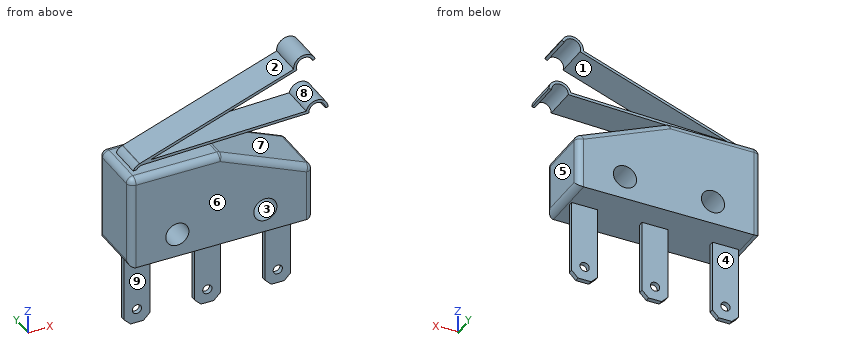
from build123d import *

# Parameters (mm, degrees)
F0_R     = 1.25
F1_DEPTH = 3.2
F2_R     = 0.7
F4_DEPTH = 1.8
F5_W     = 2.8
F5_H     = 9.0560415828
F5_R     = 0.5
F6_DEPTH = 0.25
F7_SIZE  = 0.7
F9_DEPTH = 3.6


with BuildPart() as f1:
    # F0 (on Front) → F1 (new body, symmetric)
    with BuildSketch(Plane.XZ):
        Polygon((-14.2658203304, 13.9623457611), (-24.1658203304, 13.9623457611), (-24.1658203304, 3.7623457611), (-4.3658203304, 3.7623457611), (-4.3658203304, 9.7123457611), align=None)
        with Locations((-19.0158203304, 6.2623457611)):
            Circle(F0_R, mode=Mode.SUBTRACT)
        with Locations((-9.5158203304, 6.2623457611)):
            Circle(F0_R, mode=Mode.SUBTRACT)
    extrude(amount=F1_DEPTH, both=True)

    # F2
    f2_edges = [f1.edges().sort_by_distance(p)[0] for p in [
        (-4.36582, 0, 9.712346),
        (-14.26582, 0, 13.962346),
        (-24.16582, 0, 13.962346),
        (-4.36582, 0, 3.762346),
        (-24.16582, 0, 3.762346),
        (-19.21582, -3.2, 13.962346),
        (-9.31582, -3.2, 11.837346),
        (-4.36582, -3.2, 6.737346),
        (-4.36582, 3.2, 6.737346),
        (-9.31582, 3.2, 11.837346),
        (-19.21582, 3.2, 13.962346),
        (-24.16582, -3.2, 8.862346),
        (-24.16582, 3.2, 8.862346),
    ]]
    fillet(f2_edges, radius=F2_R)

    # F3 (on Front) → F4 (join, symmetric)
    with BuildSketch(Plane.XZ):
        with BuildLine():
            Line((-4.3866957854, 15.2251207005), (-22.0158203304, 14.6623457611))
            ThreePointArc((-22.0158203304, 14.6623457611), (-23.165946247, 13.572328355), (-22.2182437598, 12.3023726214))
            Line((-22.2182437598, 12.3023726214), (-22.2182437598, 12.6108806694))
            ThreePointArc((-22.2182437598, 12.6108806694), (-22.8638430635, 13.5776541553), (-22.0062482997, 14.3624985062))
            Line((-22.0062482997, 14.3624985062), (-4.1153620949, 14.9336296691))
            ThreePointArc((-4.1153620949, 14.9336296691), (-3.2445364224, 15.8618875256), (-2.3162785659, 14.991061853))
            Line((-2.3162785659, 14.991061853), (-2.0164313111, 15.0006338837))
            ThreePointArc((-2.0164313111, 15.0006338837), (-3.1026751203, 16.1569997534), (-4.3866957854, 15.2251207005))
        make_face()
    extrude(amount=F4_DEPTH, both=True)

    # F5 (on Front) → F6 (join, symmetric)
    with BuildSketch(Plane.XZ):
        with Locations((-21.8658203304, -0.2096334475)):
            Rectangle(F5_W, F5_H)
        with Locations((-21.8658203304, -3.2376542389)):
            Circle(F5_R, mode=Mode.SUBTRACT)
        with Locations((-14.2658203304, -0.2096334475)):
            Rectangle(F5_W, F5_H)
        with Locations((-14.2658203304, -3.2376542389)):
            Circle(F5_R, mode=Mode.SUBTRACT)
        with Locations((-6.6658203304, -0.2096334475)):
            Rectangle(F5_W, F5_H)
        with Locations((-6.6658203304, -3.2376542389)):
            Circle(F5_R, mode=Mode.SUBTRACT)
    extrude(amount=F6_DEPTH, both=True)

    # F7
    f7_edges = [f1.edges().sort_by_distance(p)[0] for p in [
        (-12.86582, 0, -4.737654),
        (-15.66582, 0, -4.737654),
        (-20.46582, 0, -4.737654),
        (-23.26582, 0, -4.737654),
        (-5.26582, 0, -4.737654),
        (-8.06582, 0, -4.737654),
    ]]
    chamfer(f7_edges, length=F7_SIZE)

    # F8 (on face) → F9 (join, through all)
    with BuildSketch(Plane.XZ.offset(1.8)):
        with BuildLine():
            Line((-3.6950556462, 20.861555612), (-3.4121199517, 20.961292229))
            ThreePointArc((-3.4121199517, 20.961292229), (-4.7971701976, 21.7353058315), (-5.7393789628, 20.4587072715))
            Line((-5.7393789628, 20.4587072715), (-22.3494407238, 14.6035557305))
            Line((-22.3494407238, 14.6035557305), (-22.3988404472, 14.5861420164))
            ThreePointArc((-22.3988404472, 14.5861420164), (-23.1509491325, 13.2564048538), (-21.9777702725, 12.2778754681))
            Line((-21.9777702725, 12.2778754681), (-21.9777702725, 12.5778754681))
            ThreePointArc((-21.9777702725, 12.5778754681), (-22.8575253326, 13.319893669), (-22.2744995865, 14.3121844306))
            Line((-22.2744995865, 14.3121844306), (-5.3926698134, 20.2631359101))
            ThreePointArc((-5.3926698134, 20.2631359101), (-4.8430725807, 21.4111528446), (-3.6950556462, 20.861555612))
        make_face()
        with BuildLine():
            Line((-22.3988404472, 14.5861420164), (-22.3494407238, 14.6035557305))
            ThreePointArc((-22.3494407238, 14.6035557305), (-22.3742362034, 14.5951201251), (-22.3988404472, 14.5861420164))
        make_face()
    extrude(amount=-F9_DEPTH)


solid = f1.part
Here's how the part is built. I have some questions about the finished solid (model axes, mm). Face numbers are marked on the shaded views. A direction names the side the tool comes from. Coordinates: 2 decimals unless noted, no trailing zeros. Order: outer loops, then holes, each group sorted by start corner. A loop starts at its lowest first (then second) coordinate and runs counter-clockwise, first axis right, second up. Notation, with made-up numbers: (70.5, 45) - (79.5, 45) arc R34 cw to (79.5, 84) - close; hole circle Ø8 at (-10.5, 54). An arc over 180 degrees is marked (long way). Use CSV: the item, a comma, the result in double quotes. Start each with the question number.
1. Suppose I cut it at A-A on z = -0.5. List the corners of the cut face in (x, y) for me.
2. For the marked faces 5, 6, 7, 8 and 9, which set-ups out of +Z, -Z, +X, -X, +Y, -Y let a thin tool reach every point of the face, with its end or its side?
3. Suppose I cut it at C-C on y = -0.75. List the corners of the cut face in (x, z) for me.
4. I'm going to push flat-ended pins straight in: pin 1 (4 mm diameter, centred on x = -13.5, z = 18.5, fed in from -Y); pin 2 (6 mm diameter, centred on x = -9.5, z = 17.5, fed in from +Y); pin 3 (0.6 mm diameter, centred on y = 0, z = -1, fed in from +X); pin 4 (3 mm diameter, centred on x = -19.02, z = 6.26, fed in from -Y). Where does each tip first touch, or does it pass through?
5. Suppose I cut it at B-B on x = -18.5. List the corners of the cut face in (y, z) for me.
6. Please list where these lines run through material, in increasing order: line 1 (Z direction, x = -18, y = 0.25); line 2 (Z direction, x = -8.5, y = -1.25); line 3 (X direction, y = 0.75, z = 7). Write a range as from..to.
7. Suppose I cut it at D-D on z = 18.5. List the corners of the cut face in (x, y) for me.
8. If we mould it in two halves opening along Z, with no side actions, what happens to the marked faces 1, 2, 3 and 4? For each: +Z half, -Z half, draft (parallel to the pull), parting line (faces both ways), or undercut.
Output:
1,outline,"(-23.27, -0.25) - (-20.47, -0.25) - (-20.47, 0.25) - (-23.27, 0.25) - close; (-15.67, -0.25) - (-12.87, -0.25) - (-12.87, 0.25) - (-15.67, 0.25) - close; (-8.07, -0.25) - (-5.27, -0.25) - (-5.27, 0.25) - (-8.07, 0.25) - close"
2,face 5,"-Z, +X, +Y, -Y"
2,face 6,"+Z, -Z, +X, -X, -Y"
2,face 7,"+X, +Y, -Y"
2,face 8,"+Y, -Y"
2,face 9,"-Z, +X, -X, -Y"
3,outline,"(-24.17, 4.46) arc R0.7 ccw to (-23.47, 3.76) - (-5.07, 3.76) arc R0.7 ccw to (-4.37, 4.46) - (-4.37, 9.25) arc R0.7 ccw to (-4.79, 9.89) - (-14.13, 13.91) arc R0.7 ccw to (-14.41, 13.96) - (-22.72, 13.96) arc R0.89 cw to (-22.01, 14.36) - (-4.12, 14.93) arc R0.9 cw to (-2.32, 14.99) - (-2.02, 15) arc R1.2 ccw to (-4.39, 15.23) - (-21.21, 14.69) - (-5.39, 20.26) arc R0.9 cw to (-3.7, 20.86) - (-3.41, 20.96) arc R1.2 ccw to (-5.74, 20.46) - (-22.35, 14.6) arc R1.19 ccw to (-23.06, 13.96) - (-23.47, 13.96) arc R0.7 ccw to (-24.17, 13.26) - close; hole circle Ø2.5 at (-19.02, 6.26); hole circle Ø2.5 at (-9.52, 6.26)"
4,pin 1,"stops at y = -1.8"
4,pin 2,"stops at y = 1.8"
4,pin 3,"stops at x = -5.27"
4,pin 4,"stops at y = -3.2"
5,outline,"(-3.2, 3.76) - (3.2, 3.76) - (3.2, 5.12) - (-3.2, 5.12) - close; (-3.2, 7.4) - (3.2, 7.4) - (3.2, 13.26) arc R0.7 ccw to (2.5, 13.96) - (-2.5, 13.96) arc R0.7 ccw to (-3.2, 13.26) - close; (-1.8, 14.47) - (1.8, 14.47) - (1.8, 14.77) - (-1.8, 14.77) - close; (-1.8, 15.64) - (1.8, 15.64) - (1.8, 15.96) - (-1.8, 15.96) - close"
6,line 1,"z = 3.76..5.53, 6.99..13.96, 14.49..14.79, 15.82..16.14"
6,line 2,"z = 3.76..5.53, 6.99..11.49, 14.79..15.09, 19.17..19.49"
6,line 3,"x = -24.17..-20.02, -18.01..-10.52, -8.51..-4.37"
7,outline,"(-11.3, -1.8) - (-10.39, -1.8) - (-10.39, 1.8) - (-11.3, 1.8) - close"
8,face 1,"undercut"
8,face 2,"+Z half"
8,face 3,"undercut"
8,face 4,"draft"
